from build123d import *

# Parameters (mm, degrees)
BOSS_EXTRUDE3_DEPTH = 37.581213244
BOSS_EXTRUDE4_DEPTH = 17.71872424


with BuildPart() as part:
    # Sketch1 → Boss-Extrude3 (new body)
    with BuildSketch(Plane.XY):
        Polygon((-21.245059289, 35.57312253), (-21.245059289, -14.42687747), (28.754940711, -14.42687747), align=None)
    extrude(amount=BOSS_EXTRUDE3_DEPTH)

    # Sketch1<9> → Boss-Extrude4 (add)
    with BuildSketch(Plane.XY):
        Polygon((3.754940711, 35.57312253), (-21.245059289, 35.57312253), (3.754940711, 10.57312253), align=None)
        Polygon((28.754940711, 10.57312253), (3.754940711, 10.57312253), (28.754940711, -14.42687747), align=None)
    extrude(amount=BOSS_EXTRUDE4_DEPTH)


solid = part.part
Geometry check sheet. Reference: the model listing, model coordinates, mm. A direction names the side the tool comes from. Round coordinates to 2 decimals unless told otherwise and drop trailing zeros. Loops run counter-clockwise (first coordinate to the right, second up) from the corner with the lowest first, then second, coordinate; pieces in that order, holes last.
Item 1: Gauge pin test, flat ends, axial feed: pin 1 (8 mm diameter, centred on y = 0, z = 26.5, fed in from +X); pin 2 (19.5 mm diameter, centred on y = 20, z = 4.5, fed in from +X); pin 3 (12 mm diameter, centred on y = 16.5, z = 27.5, fed in from +X); pin 4 (9 mm diameter, centred on x = 16.5, z = 11, fed in from +Y). Record the tip position at first contact, or that the pin passes through.
Item 2: Cross-section at A-A on x = -4. Record the boundary of the cut face in (y, z), then the cut area to 3 significant figures.
Item 3: Access from +Z, -Z, +X, -X, +Y, -Y to the whole of each face (thin tool, end or side, straight path). Record for faces 1 (the flat face through (16, 10.573, 9)), 2 (the flat face through (-9, 35.573, 9)), 3 (the flat face through (-3, 29, 17.719)).
Item 4: Cross-section at C-C on y = 13. Record the boundary of the cut face in (x, z).
Item 5: Cross-section at B-B on z = 33. Record the boundary of the cut face in (x, y), then the cut area to 3 significant figures.
Item 6: Thickness scan on line 1 (X direction, y = 21.5, z = 9); line 2 (Y direction, x = 13.5, z = 16); line 3 (Z direction, x = 25.5, y = -6). Record the ranges inside material, lowest first.
Answer sheet:
1. pin 1: stops at x = 18.33
1. pin 2: stops at x = 28.75
1. pin 3: stops at x = 3.83
1. pin 4: stops at y = 10.57
2. outline: (-14.43, 0) - (35.57, 0) - (35.57, 17.72) - (18.33, 17.72) - (18.33, 37.58) - (-14.43, 37.58) - close
2. area: 1,540 mm2
3. face 1: +Z, -Z, +X, +Y
3. face 2: +Z, -Z, +X, -X, +Y
3. face 3: +Z, +X, +Y
4. outline: (-21.25, 0) - (3.75, 0) - (3.75, 17.72) - (1.33, 17.72) - (1.33, 37.58) - (-21.25, 37.58) - close
5. outline: (-21.25, -14.43) - (28.75, -14.43) - (-21.25, 35.57) - close
5. area: 1,250 mm2
6. line 1: x = -21.25 to 3.75
6. line 2: y = -14.43 to 10.57
6. line 3: z = 0 to 17.72
